Input: part model. Units: mm. Frame: model coordinates. A direction names the side the tool comes from. Round coordinates to 2 decimals unless told otherwise and drop trailing zeros. Order: outer loops, then holes, each group sorted by start corner. A loop starts at its lowest first (then second) coordinate and runs counter-clockwise, first axis right, second up. Notation, with made-up numbers: (-33, 43.25) -> (-24, 43.25) arc R14 cw to (-24, 63.25) -> close; hole circle Ø7 at (-6, 18). An arc over 180 degrees is marked (long way). Use a Markdown table: item, result.
from build123d import *

# Parameters (mm, degrees)
F1_DEPTH = 10
F2_R     = 4.55
F3_DEPTH = 10
F4_T     = -1.5


with BuildPart() as f1:
    # F0 (on Top) → F1 (new body)
    with BuildSketch(Plane.XY):
        Polygon((-15.5018547277, -8.95), (0, -17.9), (15.5018547277, -8.95), (15.5018547277, 8.95), (0, 17.9), (-15.5018547277, 8.95), align=None)
    extrude(amount=F1_DEPTH)

    # F2 (on face) → F3 (join, symmetric)
    with BuildSketch(Plane.XY.offset(10)):
        Circle(F2_R)
    extrude(amount=F3_DEPTH, both=True)

    # F4
    f4_openings = [f1.faces().sort_by_distance(p)[0] for p in [
        (0, 0, 0),
        (0, 0, 20),
    ]]
    offset(amount=F4_T, openings=f4_openings, kind=Kind.INTERSECTION)


solid = f1.part
1) Pull-direction query (Y, two-part tool) for faces 4 (the flat face through (-7.86, -13.36, 4.93)), 5 (the flat face through (6, -13, 0)), 6 (the flat face through (6.903, -12.183, 4.19)); classes: +Y half, -Y half, draft (parallel to the pull), parting line (faces both ways), or undercut.
Results found:
| item | result |
|---|---|
| face 4 | -Y half |
| face 5 | draft |
| face 6 | undercut |
2) Cut plane C-C on x = -1.5. Return loops of the section in (y, z).
Results found:
| item | result |
|---|---|
| outline | (-17.03, 0) -> (-15.3, 0) -> (-15.3, 8.5) -> (-2.66, 8.5) -> (-2.66, 20) -> (-4.3, 20) -> (-4.3, 10) -> (-17.03, 10) -> close; (2.66, 8.5) -> (15.3, 8.5) -> (15.3, 0) -> (17.03, 0) -> (17.03, 10) -> (4.3, 10) -> (4.3, 20) -> (2.66, 20) -> close |
3) Cut plane A-A on y = 0. Return loops of the section in (x, z), and give its area (3 significant figures).
Results found:
| item | result |
|---|---|
| outline | (-15.5, 0) -> (-14, 0) -> (-14, 8.5) -> (-3.05, 8.5) -> (-3.05, 20) -> (-4.55, 20) -> (-4.55, 10) -> (-15.5, 10) -> close; (3.05, 8.5) -> (14, 8.5) -> (14, 0) -> (15.5, 0) -> (15.5, 10) -> (4.55, 10) -> (4.55, 20) -> (3.05, 20) -> close |
| area | 92.9 mm² |
4) Cut plane B-B on z = 2.5. Return loops of the section in (x, y), and give its area (3 significant figures).
Results found:
| item | result |
|---|---|
| outline | (-15.5, -8.95) -> (0, -17.9) -> (15.5, -8.95) -> (15.5, 8.95) -> (0, 17.9) -> (-15.5, 8.95) -> close; hole (-14, -8.08) -> (0, -16.17) -> (14, -8.08) -> (14, 8.08) -> (0, 16.17) -> (-14, 8.08) -> close |
| area | 153 mm² |
5) Pin query (flat end, axial travel): pin 1 Ø6 at (x, y) = (6, -8) entering from +Z; pin 2 Ø2 at (x, y) = (-9.5, -9) entering from -Z; pin 3 Ø1.5 at (x, z) = (-8.5, 10) entering from +Y. Return the tip coordinate at first contact, or that it passes through.
Results found:
| item | result |
|---|---|
| pin 1 | stops at z = 10 |
| pin 2 | stops at z = 8.5 |
| pin 3 | stops at y = 13.43 |
6) Line query: L1, parallel to Y at x = 0, z = 11.25; L2, parallel to X at y = 2, z = 6.25; L3, parallel to Z at x = 8, y = -2. Output: solid intervals per line, ascending. Write a range as [from, to].
Results found:
| item | result |
|---|---|
| L1 | y = [-4.55, -3.05], [3.05, 4.55] |
| L2 | x = [-15.5, -14], [14, 15.5] |
| L3 | z = [8.5, 10] |
7) Set-up query: faces 1 (the flat face through (7.86, 13.36, 4.93)), 2 (the cylindrical face through (-0.99, -4.44, 15.07)), 3 (the flat face through (7.1, 12.07, 4.19)). Return all of +Z, -Z, +X, -X, +Y, -Y with unobstructed straight access to the full face (end or side cutting, diameter ignored); none if empty.
Results found:
| item | result |
|---|---|
| face 1 | +Z, -Z, +X, +Y |
| face 2 | +Z |
| face 3 | -Z |
8) Cut plane D-D on y = -6. Return loops of the section in (x, z).
Results found:
| item | result |
|---|---|
| outline | (-15.5, 0) -> (-14, 0) -> (-14, 8.5) -> (14, 8.5) -> (14, 0) -> (15.5, 0) -> (15.5, 10) -> (-15.5, 10) -> close |
